Can you work these out from the model? Positions are in its coordinate system, mm. A direction names the side the tool comes from. Coordinates: 2 decimals unless noted, no trailing zeros. Loops run counter-clockwise (first coordinate to the right, second up) from the corner with the lowest first, then second, coordinate; pieces in that order, holes last. Notation, with made-up numbers: M 77,51 L 132,51 A30 cw 132,74 Z; hole C 61.25,66.5 d11. An arc over 180 degrees is marked long. Answer as a JSON object with one key per item and string values. Group by question number.
Item 1: Suppose I cut it at A-A (z = 0). Write out the boundary of the cut face in (x, y).
Item 2: Suppose I cut it at B-B (x = 22.5). Write out the boundary of the cut face in (y, z), then the cut area to 3 significant figures.
Item 3: Suppose I cut it at D-D (x = 5.75). Write out the boundary of the cut face in (y, z), then the cut area to 3 significant figures.
Item 4: If I drill on line 1 (Z direction, x = 22.5, y = -195.25); line 2 (X direction, y = -30, z = 1); line 3 (Y direction, x = 16, z = -2), over which ranges is the centre line in solid material (lowest first)?
Item 5: I'm going to push flat-ended pins straight in: pin 1 Ø12 at (x, z) = (25, 6.5) entering from +Y; pin 2 Ø12 at (x, z) = (19.5, -24.5) entering from +Y. Where does each tip first touch, or does it pass through?
Item 6: We'd pull the mould along X, two halves only. Please class faces 1 (the flat face through (15, -200, 1)), 2 (the flat face through (30, -195, -1)), 3 (the cylindrical face through (20.66, -195.07, 31.19)): +X half, -X half, draft (parallel to the pull), parting line (faces both ways), or undercut.
Item 7: Which directions (+Z, -Z, +X, -X, +Y, -Y) give clear straight access to the entire face, cutting with the end or side of a thin tool? Please do faces 4 (the cylindrical face through (20.66, -195.07, -27.81)), 5 (the flat face through (22, -190, 1)).
Item 8: Suppose I cut it at C-C (y = 8). Write out the boundary of the cut face in (x, z), then the cut area to 3 significant figures.
```python
from build123d import *

# Parameters (mm, degrees)
BOSS_EXTRUDE1_DEPTH = 15
SKETCH2_W           = 15
SKETCH2_H           = 74
BOSS_EXTRUDE2_DEPTH = 10
SKETCH3_R           = 2.5
CUT_EXTRUDE1_DEPTH  = 10
SKETCH4_R           = 11
CUT_EXTRUDE2_DEPTH  = 31


with BuildPart() as part:
    # Sketch1 → Boss-Extrude1 (new body)
    with BuildSketch(Plane(origin=(0, 0, 0), x_dir=(0, 0, -1), z_dir=(1, 0, 0))):
        with BuildLine():
            Line((-37, 0), (-37, -200))
            Line((-37, -200), (37, -200))
            Line((37, -200), (37, 0))
            ThreePointArc((37, 0), (0, 37), (-37, 0))
        make_face()
    extrude(amount=BOSS_EXTRUDE1_DEPTH)

    # Sketch2 → Boss-Extrude2 (add)
    with BuildSketch(Plane.XZ.offset(200)):
        with Locations((22.5, 0)):
            Rectangle(SKETCH2_W, SKETCH2_H)
    extrude(amount=-BOSS_EXTRUDE2_DEPTH)

    # Sketch3 → Cut-Extrude1 (cut)
    with BuildSketch(Plane.XZ.offset(200)):
        with Locations((22.5, 29.5)):
            Circle(SKETCH3_R)
        with Locations((22.5, -29.5)):
            Circle(SKETCH3_R)
    extrude(amount=-CUT_EXTRUDE1_DEPTH, mode=Mode.SUBTRACT)

    # Sketch4 → Cut-Extrude2 (cut, through all)
    with BuildSketch(Plane.ZY):
        Circle(SKETCH4_R)
    extrude(amount=-CUT_EXTRUDE2_DEPTH, mode=Mode.SUBTRACT)


solid = part.part
```
From the geometry:
{
 "1": {"outline": "M 0,-200 L 30,-200 L 30,-190 L 15,-190 L 15,-11 L 0,-11 Z; M 0,11 L 15,11 L 15,37 L 0,37 Z"},
 "2": {"outline": "M -200,-37 L -190,-37 L -190,-32 L -200,-32 Z; M -200,-27 L -190,-27 L -190,27 L -200,27 Z; M -200,32 L -190,32 L -190,37 L -200,37 Z", "area": "640 mm2"},
 "3": {"outline": "M -200,-37 L 0,-37 A37 ccw 0,37 L -200,37 Z; hole C 0,0 d22", "area": "16,600 mm2"},
 "4": {"line 1": "-37 to -32, -27 to 27, 32 to 37", "line 2": "0 to 15", "line 3": "-200 to -190"},
 "5": {"pin 1": "y = -190", "pin 2": "y = 30.78"},
 "6": {"face 1": "draft", "face 2": "+X half", "face 3": "undercut"},
 "7": {"face 4": "+Y, -Y", "face 5": "+Z, -Z, +X, +Y"},
 "8": {"outline": "M 0,-36.12 L 15,-36.12 L 15,-7.55 L 0,-7.55 Z; M 0,7.55 L 15,7.55 L 15,36.12 L 0,36.12 Z", "area": "857 mm2"}
}
